```python
from build123d import *

# Parameters (mm, degrees)
SKETCH2_R          = 3.175
CUT_EXTRUDE1_DEPTH = 17.228257088
CHAMFER1_SIZE      = 0.508


with BuildPart() as part:
    # Sketch1 → Revolve1 (revolve)
    with BuildSketch(Plane(origin=(0, 0, 0), x_dir=(0, 0, -1), z_dir=(1, 0, 0)), mode=Mode.PRIVATE) as revolve1_sk:
        Polygon((0, 0), (0, 7.14375), (1.5875, 7.14375), (1.5875, 5.4689375), (1.4843125, 5.4689375), (1.4843125, 5.0561875), (1.8970625, 5.0561875), (1.8970625, 5.159375), (12.7, 5.159375), (12.7, 0), align=None)
    revolve(revolve1_sk.sketch.rotate(Axis((0, 0, 0), (0, 0, 1)), 90), axis=Axis((0, 0, 0), (0, 0, 1)))

    # Sketch2 → Cut-Extrude1 (cut, through all)
    with BuildSketch(Plane.XY):
        Circle(SKETCH2_R)
    extrude(amount=-CUT_EXTRUDE1_DEPTH, mode=Mode.SUBTRACT)

    # Chamfer1
    chamfer1_edges = [part.edges().sort_by_distance(p)[0] for p in [
        (5.159375, 0, -12.7),
    ]]
    chamfer(chamfer1_edges, length=CHAMFER1_SIZE)


solid = part.part
```
CAD build for the part. Positions are in the model's coordinates, mm. A direction names the side the tool comes from. Coordinates: 2 decimals unless noted, no trailing zeros. Order: outer loops, then holes, each group sorted by start corner. A loop starts at its lowest first (then second) coordinate and runs counter-clockwise, first axis right, second up.
(1) Which spindle directions (+Z, -Z, +X, -X, +Y, -Y) get a long thin tool onto all of the face, cutting with end or side? Do faces 1 (the face through (7.137, -0.314, -0.805)), 2 (the face through (-4, 4, -1.588)). Say none if no direction does.
Solution:
face 1: +Z, -Z
face 2: -Z
(2) Saw through at D-D, the plane y = 6. Write the cut outline in (x, z), and give its area (3 significant figures).
Solution:
outline: (-3.88, -1.59) - (3.88, -1.59) - (3.88, 0) - (-3.88, 0) - close
area: 12.3 mm2
(3) Pin check, flat tips, straight feed: pin 1 Ø3 at (x, z) = (0.5, -7.5) entering from -Y; pin 2 Ø2 at (y, z) = (5.5, -3) entering from +X; pin 3 Ø5 at (x, y) = (0, 0) entering from +Z; pin 4 Ø2 at (y, z) = (3.5, -10.5) entering from +X. Stop position of each tip, or through.
Solution:
pin 1: stops at y = -5.16
pin 2: stops at x = 2.52
pin 3: passes through
pin 4: stops at x = 4.51
(4) Saw through at C-C, the plane z = -4. Write the cut outline in (x, y) (3 decimals), and give its area (3 significant figures).
Solution:
outline: circle Ø10.319 at (0, 0); hole circle Ø6.35 at (0, 0)
area: 52.0 mm2
(5) Mould opens along Z. For faces 3 (the face through (-0.69, -3.1, -6.26)), 4 (the face through (3.1, 1.5, 0)), 5 (the face through (-2, 3, -12.7)), 6 (the face through (1.096, 4.936, -1.694)) say: released by +Z, released by -Z, zero draft, split by the parting line, or undercut.
Solution:
face 3: zero draft
face 4: released by +Z
face 5: released by -Z
face 6: undercut
(6) Drill centre lines: L1, parallel to Y at x = 0, z = -1.55 (3 decimals); L2, parallel to Y at x = 0, z = -9 (3 decimals); L3, parallel to Y at x = 0, z = -1.45 (3 decimals). Where is each one in solid material? Low to high.
Solution:
L1: y = -7.144 to -5.469, -5.056 to -3.175, 3.175 to 5.056, 5.469 to 7.144
L2: y = -5.159 to -3.175, 3.175 to 5.159
L3: y = -7.144 to -3.175, 3.175 to 7.144
